from build123d import *

# Parameters (mm, degrees)
CYLINDER003005_R          = 1.7
CYLINDER003005_DEPTH      = 10
CYLINDER002010_R          = 3.5
CYLINDER002010_DEPTH      = 16
BOX001001007_W            = 1.5
BOX001001007_H            = 0.25
BOX001001007_DEPTH        = 4.6
BOX001001008_W            = 1.5
BOX001001008_H            = 0.25
BOX001001008_DEPTH        = 4.6
BOX001001_W               = 1.5
BOX001001_H               = 0.25
BOX001001_DEPTH           = 4.6
BOX001001_PLACEMENT_ANGLE = 90
BOX001002_W               = 1.5
BOX001002_H               = 0.25
BOX001002_DEPTH           = 4.6
BOX001002_PLACEMENT_ANGLE = 90
CYLINDER004013_R          = 5
CYLINDER004013_DEPTH      = 1.5
CHAMFER009_SIZE           = 0.5
CYLINDER001009_R          = 4
CYLINDER001009_DEPTH      = 4.6
CUT003013_ROLL_ANGLE      = -90


with BuildPart() as hole:
    # Cylinder003005 → Cylinder003005 (new body)
    with BuildSketch(Plane.XY.offset(-8)):
        Circle(CYLINDER003005_R)
    extrude(amount=CYLINDER003005_DEPTH)


with BuildPart() as cylinder002010:
    # Cylinder002010 → Cylinder002010 (new body)
    with BuildSketch(Plane.XY.offset(-14.5)):
        Circle(CYLINDER002010_R)
    extrude(amount=CYLINDER002010_DEPTH)


with BuildPart() as contact:
    # Box001001007 → Box001001007 (new body)
    with BuildSketch(Plane(origin=(-1, -3, -19), x_dir=(1, 0, 0), z_dir=(0, 0, 1))):
        with Locations((0.75, 0.125)):
            Rectangle(BOX001001007_W, BOX001001007_H)
    extrude(amount=BOX001001007_DEPTH)


with BuildPart() as contact001:
    # Box001001008 → Box001001008 (new body)
    with BuildSketch(Plane(origin=(-1, 2, -19), x_dir=(1, 0, 0), z_dir=(0, 0, 1))):
        with Locations((0.75, 0.125)):
            Rectangle(BOX001001008_W, BOX001001008_H)
    extrude(amount=BOX001001008_DEPTH)


with BuildPart() as contact002:
    # Box001001 → Box001001 (new body)
    with BuildSketch(Plane.XY):
        with Locations((0.75, 0.125)):
            Rectangle(BOX001001_W, BOX001001_H)
    extrude(amount=BOX001001_DEPTH)


with BuildPart() as contact002_1:
    # Box001001 placement: moved
    add(contact002.part.moved(Location((2, -0.8, -19))).rotate(Axis((2, -0.8, -19), (0, 0, 1)), BOX001001_PLACEMENT_ANGLE))


with BuildPart() as contact003:
    # Box001002 → Box001002 (new body)
    with BuildSketch(Plane.XY):
        with Locations((0.75, 0.125)):
            Rectangle(BOX001002_W, BOX001002_H)
    extrude(amount=BOX001002_DEPTH)


with BuildPart() as contact003_1:
    # Box001002 placement: moved
    add(contact003.part.moved(Location((-2, -0.9, -19))).rotate(Axis((-2, -0.9, -19), (0, 0, 1)), BOX001002_PLACEMENT_ANGLE))


with BuildPart() as chamfer009:
    # Cylinder004013 → Cylinder004013 (new body)
    with BuildSketch(Plane.XY):
        Circle(CYLINDER004013_R)
    extrude(amount=CYLINDER004013_DEPTH)

    # Chamfer009
    chamfer009_edges = [chamfer009.edges().sort_by_distance(p)[0] for p in [
        (-5, 0, 1.5),
    ]]
    chamfer(chamfer009_edges, length=CHAMFER009_SIZE)


with BuildPart() as f_4_way_jack_socket:
    # Cylinder001009 → Cylinder001009 (new body)
    with BuildSketch(Plane.XY.offset(-4.5)):
        Circle(CYLINDER001009_R)
    extrude(amount=CYLINDER001009_DEPTH)

    # Fusion001002: union Cylinder002010, Contact, Contact001, Contact002, Contact003, Chamfer009
    add(cylinder002010.part)
    add(contact.part)
    add(contact001.part)
    add(contact002_1.part)
    add(contact003_1.part)
    add(chamfer009.part)

    # Cut003013: cut hole
    add(hole.part, mode=Mode.SUBTRACT)


with BuildPart() as f_4_way_jack_socket_1:
    # Cut003013 roll: moved
    add(f_4_way_jack_socket.part.rotate(Axis((0, 0, 0), (1, 0, 0)), CUT003013_ROLL_ANGLE))


with BuildPart() as f_4_way_jack_socket_2:
    # Cut003013 placement: moved
    add(f_4_way_jack_socket_1.part.moved(Location((12.5, 32, 60))))


solid = f_4_way_jack_socket_2.part
For this review, take the finished solid that the model builds, in its own axes (mm). A direction names the side the tool comes from. Round coordinates to 2 decimals unless told otherwise and drop trailing zeros. Write each loop counter-clockwise with the first axis right and the second up, starting at its lowest first coordinate (ties: lowest second). Pieces come first, ordered by that corner, then holes. Notation, with made-up numbers: (15.25, -5) -> (28.25, -5) arc R29 ccw to (28.25, 29) -> close; hole circle Ø5 at (-14, 10.5). An arc over 180 degrees is marked (long way). Put each result on its own line as item: value.
Q1. Consider section C-C on x = 12.5. State the section outline as (y, z) points, and give its area (3 significant figures).
Determined:
outline: (13, 57.75) -> (17.5, 57.75) -> (17.5, 56.5) -> (27.5, 56.5) -> (27.5, 56) -> (32, 56) -> (32, 55) -> (33, 55) -> (33.5, 55.5) -> (33.5, 58.3) -> (24, 58.3) -> (24, 61.7) -> (33.5, 61.7) -> (33.5, 64.5) -> (33, 65) -> (32, 65) -> (32, 64) -> (27.5, 64) -> (27.5, 63.5) -> (17.5, 63.5) -> (17.5, 63) -> (13, 63) -> (13, 62.75) -> (17.5, 62.75) -> (17.5, 58) -> (13, 58) -> close
area: 90.7 mm^2
Q2. To check wall thickness, follow L1, parallel to X at y = 29, z = 60; L2, parallel to Z at x = 12.5, y = 29.25; L3, parallel to Z at x = 12.5, y = 26.75. State the ranges of each line that lie inside material, in increasing order. Write a range as [from, to].
Determined:
L1: x = [8.5, 10.8], [14.2, 16.5]
L2: z = [56, 58.3], [61.7, 64]
L3: z = [56.5, 58.3], [61.7, 63.5]
Q3. The part is to be moulded in two halves that separate along Z. For faces 1 (the flat face through (12, 15, 62.75)), 2 (the flat face through (12, 15, 63)), 3 (the flat face through (14.25, 15, 60)), say which applies: released by +Z, released by -Z, zero draft, split by the parting line, or undercut.
Determined:
face 1: undercut
face 2: released by +Z
face 3: zero draft
Q4. Consider section A-A on y = 16.25. State the section outline as (x, z) points, and give its area (3 significant figures).
Determined:
outline: (10.25, 59.4) -> (10.5, 59.4) -> (10.5, 60.9) -> (10.25, 60.9) -> close; (11.5, 57.75) -> (13, 57.75) -> (13, 58) -> (11.5, 58) -> close; (11.5, 62.75) -> (13, 62.75) -> (13, 63) -> (11.5, 63) -> close; (14.25, 59.3) -> (14.5, 59.3) -> (14.5, 60.8) -> (14.25, 60.8) -> close
area: 1.50 mm^2
Q5. Machinability: for faces 4 (the flat face through (12, 15, 57.75)), 5 (the flat face through (10.25, 15, 60)), 6 (the flat face through (10.5, 15, 60)), which of the approach directions +Z, -Z, +X, -X, +Y, -Y give a long, thin tool a straight path to every point of the face, cutting with its end or side? Answer none if there is none.
Determined:
face 4: -Z, +X, -X, -Y
face 5: +Z, -Z, -X, -Y
face 6: +Z, -Z, -Y
Q6. Clearance check with flat-ended pins moving along their axes: pin 1 Ø3 at (y, z) = (28, 60.5) entering from +X; pin 2 Ø6 at (x, y) = (16, 31) entering from +Z; pin 3 Ø3 at (x, z) = (14, 62.5) entering from -Y; pin 4 Ø1.6 at (x, y) = (12, 15.5) entering from +Z. State where each tip first meets the part, or that it passes through.
Determined:
pin 1: stops at x = 16.5
pin 2: stops at z = 64.95
pin 3: stops at y = 13
pin 4: stops at z = 63
Q7. Consider section B-B on z = 60. State the section outline as (x, y) points, and give its area (3 significant figures).
Determined:
outline: (7.5, 32) -> (8.5, 32) -> (8.5, 27.5) -> (9, 27.5) -> (9, 17.5) -> (10.25, 17.5) -> (10.25, 13) -> (10.5, 13) -> (10.5, 17.5) -> (14.25, 17.5) -> (14.25, 13) -> (14.5, 13) -> (14.5, 17.5) -> (16, 17.5) -> (16, 27.5) -> (16.5, 27.5) -> (16.5, 32) -> (17.5, 32) -> (17.5, 33) -> (17, 33.5) -> (14.2, 33.5) -> (14.2, 24) -> (10.8, 24) -> (10.8, 33.5) -> (8, 33.5) -> (7.5, 33) -> close
area: 90.7 mm^2
